Autodesk Inventor part; units mm, degrees
ref_plane "YZ Plane" through (0, 0, 0) normal (1, 0, 0) x (0, 1, 0)
ref_plane "XZ Plane" through (0, 0, 0) normal (0, 1, 0) x (-1, 0, 0)
ref_plane "XY Plane" through (0, 0, 0) normal (0, 0, 1) x (1, 0, 0)
sketch "Sketch1" plane through (0, 0, 0) normal (0, 0, 1) x (1, 0, 0)
  circle A0 centre (0, 0) radius 15.875
  line L0 (0, 15.875) -> (0, 25.4)
  line L1 (0, 25.4) -> (-30.5689, 25.4)
  line L2 (-30.5689, 25.4) -> (-30.5689, -25.4)
  line L3 (-30.5689, -25.4) -> (0, -25.4)
  line L4 (0, -25.4) -> (0, -15.875)
  line L5 (0, -15.875) -> (0, 15.875)
  line L6 (0, 25.4) -> (45.6311, 25.4)
  line L7 (45.6311, 25.4) -> (45.6311, -25.4)
  line L8 (45.6311, -25.4) -> (0, -25.4)
  line L9 (0, -25.4) -> (0, 25.4)
  line L10 (7.5311, 25.4) -> (7.5311, -25.4) construction
  line L11 (-17.8689, 25.4) -> (-17.8689, -25.4) construction
  line L12 (32.9311, 25.4) -> (32.9311, -25.4) construction
  dimension "d0" = 31.75
  dimension "d1" = 50.8
  dimension "d3" = 7.5311
  dimension "d6" = 38.1
  dimension "d7" = 38.1
  dimension "d8" = 25.4
  dimension "d9" = 25.4
extrude "Extrusion1" add sketch "Sketch1" along normal blind 6.35 contours A0 L0 L6 L7 L8 L4 | A0 L4 L3 L2 L1 L0
chamfer "Chamfer1" distance 6.35 distance2 6.35 1 edges at (-15.875, 0, 0) measured on face at (15.8235, -1.2774, 4.2333)
sketch "Sketch2" plane through (-30.5689, -25.4, 0) normal (-1, 0, 0) x (0, 0, 1)
  line L0 (0, 0) -> (6.35, 0)
  line L1 (6.35, 0) -> (-25.4, 0)
  line L2 (-25.4, 0) -> (-25.4, -3.175)
  line L3 (-25.4, -3.175) -> (6.35, -3.175)
  line L4 (6.35, -3.175) -> (6.35, 0)
  line L5 (6.35, 50.8) -> (-25.4, 50.8)
  line L6 (-25.4, 50.8) -> (-25.4, 53.975)
  line L7 (-25.4, 53.975) -> (6.35, 53.975)
  line L8 (6.35, 53.975) -> (6.35, 50.8)
  line L9 (0, 50.8) -> (0, 0)
  point P0 (0, 25.4)
  dimension "d15" = 3.175
  dimension "d16" = 25.4
extrude "Extrusion2" add sketch "Sketch2" against normal up to surface (76.2 mm away)
sketch "Sketch3" plane through (-30.5689, 28.575, 6.35) normal (0, 1, 0) x (1, 0, 0)
  line L0 (0, 0) -> (0, 31.75)
  line L1 (0, 31.75) -> (76.2, 31.75)
  point P0 (30.5689, 6.35)
  point P1 (12.7, 19.05)
  point P2 (38.1, 19.05)
  point P3 (63.5, 19.05)
  dimension "d19" = 12.7
  dimension "d20" = 25.4
  dimension "d21" = 25.4
  dimension "d22" = 12.7
hole "Hole1" at (-17.8689, 28.575, -12.7) at (7.5311, 28.575, -12.7) at (32.9311, 28.575, -12.7) direction (0, -1, 0) diameter 4.445 end through all
sketch "Sketch4" plane through (0, 0, 0) normal (0, 0, -1) x (-1, 0, 0)
  line L0 (22.225, -15.875) -> (-22.225, -15.875)
  line L1 (-22.225, -15.875) -> (-22.225, 15.875)
  line L2 (-22.225, 15.875) -> (22.225, 15.875)
  line L3 (22.225, 15.875) -> (22.225, -15.875)
  line L4 (22.225, -15.875) -> (-22.225, 15.875) construction
  line L5 (-22.225, -15.875) -> (22.225, 15.875) construction
  circle A0 centre (0, 0) radius 15.875
  circle A1 centre (0, 0) radius 22.225
  point P0 (15.5543, 15.875)
  point P1 (-15.5543, 15.875)
  point P2 (-15.5543, -15.875)
  point P3 (15.5543, -15.875)
extrude "Extrusion3" add sketch "Sketch4" against normal up to surface (6.35 mm away) contours A1 L0 | L2 A1
sketch "Sketch5" plane through (0, 0, 6.35) normal (0, 0, 1) x (1, 0, 0)
  circle A0 centre (0, -1.5875) radius 25.0825 construction
  line L0 (-17.736, -19.3235) -> (17.736, 16.1485) construction
  line L1 (-17.736, 16.1485) -> (17.736, -19.3235) construction
  line L2 (-17.736, -19.3235) -> (17.736, -19.3235) construction
  point P0 (0, 0)
  point P1 (0, -1.5875)
  dimension "d32" = 1.5875
  dimension "d34" = 50.165
hole "Hole2" at (-17.736, -19.3235, 6.35) at (17.736, 16.1485, 6.35) at (-17.736, 16.1485, 6.35) at (17.736, -19.3235, 6.35) direction (0, 0, -1) diameter 4.572 end through all
properties part number "Inner Channel Guide"
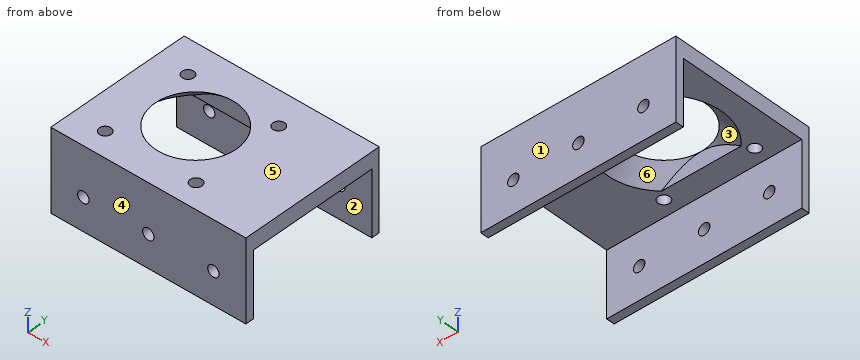
Could you check a few things on this model? Use its own coordinates, in mm. Face numbers are marked on the shaded views. A direction names the side the tool comes from. Coordinates: 2 decimals unless noted, no trailing zeros. Order: outer loops, then holes, each group sorted by start corner. A loop starts at its lowest first (then second) coordinate and runs counter-clockwise, first axis right, second up. Notation, with made-up numbers: M 70,36 L 103,36 A23 ccw 103,70 Z; hole C 25.5,86 d6. An arc over 180 degrees is marked long. Use one line per item in the form item = value. Start each with the question number.
1. Suppose I cut it at A-A on z = -18.5. Write out the boundary of the cut face in (x, y) (3 decimals).
2. Suppose I cut it at D-D on x = 40. Write out the boundary of the cut face in (y, z) (3 decimals).
3. We'd pull the mould along Y, two halves only. Please class the marked faces 4, 5 and 6: +Y half, -Y half, draft (parallel to the pull), parting line (faces both ways), or undercut.
4. For pin 1 (8 mm diameter, centred on x = -9, y = -13.5, fed in from -Z), with a flat end and sliding along its axis, tell me the tip position at first contact or that it passes through.
5. Please list where these lines run through material, in increasing order: line 1 (Y direction, x = 12, z = 0.5) (3 decimals); line 2 (Y direction, x = 32, z = -10.5) (3 decimals); line 3 (Y direction, x = -16, z = 1) (3 decimals).
6. Suppose I cut it at B-B on z = -12.7. Count the separate pieces of the cut face and the enclosed holes in it, then the cut area to 3 significant figures.
7. On a 3-axis mill with a long thin cutter (end or side, diameter ignored), from which of +Z, -Z, +X, -X, +Y, -Y can I reach the whole of each face in a straight line? I mean the marked faces 1, 2 and 3. Say none if no direction works.
Geometry says:
q1.outline = M -30.569,-28.575 L 45.631,-28.575 L 45.631,-25.4 L -30.569,-25.4 Z; M -30.569,25.4 L 45.631,25.4 L 45.631,28.575 L -30.569,28.575 Z
q2.outline = M -28.575,-25.4 L -25.4,-25.4 L -25.4,0 L 25.4,0 L 25.4,-25.4 L 28.575,-25.4 L 28.575,6.35 L -28.575,6.35 Z
q3.face_4 = -Y half
q3.face_5 = draft
q3.face_6 = undercut
q4.pin_1 = 0
q5.line_1 = -28.575 to -15.875, 15.875 to 28.575
q5.line_2 = -28.575 to -25.4, 25.4 to 28.575
q5.line_3 = -28.575 to -20.811, -17.836 to -13.946, 13.946 to 14.661, 17.636 to 28.575
q6.separate_pieces = 8
q6.enclosed_holes = 0
q6.area = 399 mm^2
q7.face_1 = +Z, -Z, +X, -X, +Y
q7.face_2 = -Z, +X, -X
q7.face_3 = -Z
